```python
from build123d import *

# Parameters (mm, degrees)
ESBO_O1_R                     = 1.65
RESSALTO_EXTRUS_O1_DEPTH      = 37.6
RESSALTO_EXTRUS_O2_DEPTH      = 2
RESSALTO_EXTRUS_O2_DEPTH_BACK = 39.6
CORTE_EXTRUS_O1_DEPTH         = 41.164163131
CORTE_EXTRUS_O1_DEPTH_BACK    = 41.164163131
ESBO_O2_W                     = 6.8
ESBO_O2_H                     = 3


with BuildPart() as part:
    # Esboço1 → Ressalto-extrusão1 (new body)
    with BuildSketch(Plane.XY):
        with BuildLine():
            Line((-5.196152423, -3), (5.196152423, -3))
            ThreePointArc((5.196152423, -3), (6, 0), (5.196152423, 3))
            Line((5.196152423, 3), (-5.196152423, 3))
            ThreePointArc((-5.196152423, 3), (-6, 0), (-5.196152423, -3))
        make_face()
        Circle(ESBO_O1_R, mode=Mode.SUBTRACT)
    extrude(amount=RESSALTO_EXTRUS_O1_DEPTH)

    # Esboço3 → Ressalto-extrusão2 (add, two sides: drawn at the far end of the back side and taken through both)
    with BuildSketch(Plane(origin=(0, 0, 0), x_dir=(-1, 0, 0), z_dir=(0, 0, -1)).offset(-RESSALTO_EXTRUS_O2_DEPTH_BACK)):
        with BuildLine():
            Line((0.8, 1.5), (5.809475019, 1.5))
            ThreePointArc((5.809475019, 1.5), (6, 0), (5.809475019, -1.5))
            Line((5.809475019, -1.5), (0.8, -1.5))
            ThreePointArc((0.8, -1.5), (1.7, 0), (0.8, 1.5))
        make_face()
        with BuildLine():
            Line((-5.809475019, 1.5), (-0.8, 1.5))
            ThreePointArc((-0.8, 1.5), (-1.7, 0), (-0.8, -1.5))
            Line((-0.8, -1.5), (-5.809475019, -1.5))
            ThreePointArc((-5.809475019, -1.5), (-6, 0), (-5.809475019, 1.5))
        make_face()
    extrude(amount=RESSALTO_EXTRUS_O2_DEPTH + RESSALTO_EXTRUS_O2_DEPTH_BACK)

    # Esboço2 → Corte-extrusão1 (cut, two sides: drawn at the far end of the back side and taken through both)
    with BuildSketch(Plane(origin=(0, 0, 0), x_dir=(1, 0, 0), z_dir=(0, 1, 0)).offset(-CORTE_EXTRUS_O1_DEPTH_BACK)):
        with Locations((0, -5.5)):
            Rectangle(ESBO_O2_W, ESBO_O2_H)
        with Locations((0, -5.5)):
            Rectangle(ESBO_O2_W, ESBO_O2_H)
        with Locations((0, -32.1)):
            Rectangle(ESBO_O2_W, ESBO_O2_H)
        with Locations((0, -32.1)):
            Rectangle(ESBO_O2_W, ESBO_O2_H)
    extrude(amount=CORTE_EXTRUS_O1_DEPTH + CORTE_EXTRUS_O1_DEPTH_BACK, mode=Mode.SUBTRACT)


solid = part.part
```
Build history of the part. All positions in model axes, mm. A direction names the side the tool comes from. Give positions to 0.01 mm unless a question says otherwise; leave off trailing zeros. Loops run counter-clockwise (first coordinate to the right, second up) from the corner with the lowest first, then second, coordinate; pieces in that order, holes last. Notation, with made-up numbers: (-25.5, 65.5) -> (4.5, 65.5) arc R15 cw to (4.5, 81.5) -> close; hole circle Ø10 at (-5, 46). An arc over 180 degrees is marked (long way). One line per question, with ' | ' between items.
Q1. Tool access for faces 4 (the flat face through (-3, -1.5, -1)), 5 (the cylindrical face through (1.7, 0, 38.6)), 6 (the cylindrical face through (-1.7, 0, -1)), 7 (the flat face through (3.4, 0, 32)), 8 (the flat face through (-3, -1.5, 39)): list every direction of +Z, -Z, +X, -X, +Y, -Y with a clear straight run to the whole face (end or side of a thin tool).
Filled sheet:
face 4: -Z, +X, -X, -Y | face 5: +Z | face 6: -Z | face 7: +Y, -Y | face 8: +Z, +X, -X, -Y
Q2. Pull direction Y, two halves, no side cores. Call faces 1 (the cylindrical face through (-1.7, 0, 38.6)), 2 (the flat face through (-2, -1, 7)), 3 (the flat face through (0, -3, 19)): pulls with the +Y half, pulls with the -Y half, needs draft (parallel to the pull), parting line crosses it, or undercut.
Filled sheet:
face 1: undercut | face 2: needs draft | face 3: pulls with the -Y half
Q3. Cut at B-B, the plane z = 24.5. Write the cut outline in (x, y), plus the area to 3 significant figures.
Filled sheet:
outline: (-5.2, -3) -> (5.2, -3) arc R6 ccw to (5.2, 3) -> (-5.2, 3) arc R6 ccw to start; hole circle Ø3.3 at (0, 0) | area: 60.3 mm²
Q4. Drop flat-ended pins along their axis: pin 1 (3 mm diameter, centred on x = 0.5, y = 1, fed in from +Z); pin 2 (0.6 mm diameter, centred on x = 3.5, z = 38.5, fed in from -Y); pin 3 (1.5 mm diameter, centred on x = 0, y = 1, fed in from +Z); pin 4 (1 mm diameter, centred on x = -4, z = 38.5, fed in from +Y). Give the stop position or say it passes through.
Filled sheet:
pin 1: stops at z = 39.6 | pin 2: stops at y = -1.5 | pin 3: stops at z = 37.6 | pin 4: stops at y = 1.5
Q5. Drill centre lines: line 1 along Z through (x, y) = (2.75, -0.25); line 2 along Z through (x, y) = (2.5, 2.5); line 3 along X through (y, z) = (0, 14). Where is each one in solid material? Low to high. Write a range as [from, to].
Filled sheet:
line 1: z = [-2, 4], [7, 30.6], [33.6, 39.6] | line 2: z = [0, 4], [7, 30.6], [33.6, 37.6] | line 3: x = [-6, -1.65], [1.65, 6]
Q6. Cut at D-D, the plane x = 0. Write the cut outline in (y, z).
Filled sheet:
outline: (-3, 0) -> (-1.65, 0) -> (-1.65, 4) -> (-3, 4) -> close; (-3, 7) -> (-1.65, 7) -> (-1.65, 30.6) -> (-3, 30.6) -> close; (-3, 33.6) -> (-1.65, 33.6) -> (-1.65, 37.6) -> (-3, 37.6) -> close; (1.65, 0) -> (3, 0) -> (3, 4) -> (1.65, 4) -> close; (1.65, 7) -> (3, 7) -> (3, 30.6) -> (1.65, 30.6) -> close; (1.65, 33.6) -> (3, 33.6) -> (3, 37.6) -> (1.65, 37.6) -> close
Q7. Cut at A-A, the plane x = 2.5. Write the cut outline in (y, z).
Filled sheet:
outline: (-3, 0) -> (-1.5, 0) -> (-1.5, -2) -> (1.5, -2) -> (1.5, 0) -> (3, 0) -> (3, 4) -> (-3, 4) -> close; (-3, 7) -> (3, 7) -> (3, 30.6) -> (-3, 30.6) -> close; (-3, 33.6) -> (3, 33.6) -> (3, 37.6) -> (1.5, 37.6) -> (1.5, 39.6) -> (-1.5, 39.6) -> (-1.5, 37.6) -> (-3, 37.6) -> close
